Build history of the part. All positions in model axes, mm. A direction names the side the tool comes from. Coordinates: 2 decimals unless noted, no trailing zeros. Write each loop counter-clockwise with the first axis right and the second up, starting at its lowest first coordinate (ties: lowest second). Pieces come first, ordered by that corner, then holes.
Autodesk Inventor part; units mm, degrees
ref_plane "Work Plane1" through (29, 0, 0) normal (0, -1, 0) x (1, 0, 0)
ref_plane "YZ Plane" through (0, 0, 0) normal (1, 0, 0) x (0, 1, 0)
ref_plane "XZ Plane" through (0, 0, 0) normal (0, 1, 0) x (-1, 0, 0)
sketch "Эскиз1" plane through (0, 0, 0) normal (0, 0, 1) x (1, 0, 0)
  line L0 (-0.7333, 0) -> (16, 0)
  line L1 (16, 0) -> (16, 1.25)
  line L2 (16, 1.25) -> (1.35, 1.25)
  line L3 (1.35, 1.25) -> (1.0738, 1.25)
  line L4 (1.0738, 1.25) -> (0, 1.25)
  line L5 (0, 1.25) -> (0, 2.25)
  line L6 (0, 2.25) -> (-2.5, 2.25)
  line L7 (-2.5, 2.25) -> (-2.5, 1.1547)
  line L8 (-2.5, 1.1547) -> (-1.4, 1.1547)
  line L9 (-1.4, 1.1547) -> (-0.7333, 0)
  line L10 (-6.2, 0) -> (19.7, 0)
  line L11 (0, -0.45) -> (0, 2.7)
  line L12 (1.35, 1.25) -> (0, 1.25) construction
  dimension "d1" = 14.65
  dimension "d2" = 0.2762
  dimension "d3" = 2.5
  dimension "d4" = 1.1
  dimension "d5" = 60
  dimension "d6" = 2.5
  dimension "d7" = 2.5
  dimension "d8" = 2.3094
  dimension "d9" = 4.5
  dimension "d26" = 16
revolve "Базовый элемент" add sketch "Эскиз1" angle 360 about axis through (-0.7333, 0, 0) along (1, 0, 0)
sketch "Эскиз2" plane through (-2.5, 0, 0) normal (-1, 0, 0) x (0, 0, 1)
  circle A0 centre (0, 0) radius 1.1547
  line L0 (0, -3.15) -> (0, 3.15)
  line L1 (-3.15, 0) -> (3.15, 0)
  line L2 (1.1547, 0) -> (0.5774, -1)
  line L3 (0.5774, -1) -> (-0.5774, -1)
  line L4 (-0.5774, -1) -> (-1.1547, 0)
  line L5 (-1.1547, 0) -> (-0.5774, 1)
  line L6 (-0.5774, 1) -> (0.5774, 1)
  line L7 (0.5774, 1) -> (1.1547, 0)
extrude "Паз" add sketch "Эскиз2" against normal up to next contours L7 A0 | A0 L2 | L6 L0 A0 | A0 L0 L3 | L0 L6 A0 | A0 L3 L0 | L4 A0 | A0 L5
fillet "Сопряжение1" radius 0.25 1 edges at (-2.5, -2.25, 0)
thread "Резьба"
chamfer "Фаска1" distance 0.2761 distance2 0.2761 1 edges at (16, -1.25, 0) measured on face at (16, -0.3871, -0.3429)
ref_plane "Work Plane1" through (29, 0, 0) normal (0, -1, 0) x (1, 0, 0)
fillet "Fillet2" radius 0.1 1 edges at (0, -1.25, 0)
equation "\"d1\" = GEL"
equation "\"d3\" = KOH"
equation "\"d4\" = INTI"
equation "\"d6\" = GD"
equation "\"d7\" = BDM"
equation "\"d8\" = 1.1547 * SW"
equation "\"d9\" = KOD"
equation "\"d26\" = NLG"
equation "\"d30\" = R"
equation "\"d17\" = RR"
equation "\"d13\" = GEL"
equation "\"d15\" = -0.5 * SPD + 0.5 * GD"
equation "\"d16\" = GUL"
equation "\"GD\" = 2.5"
equation "\"NLG\" = 16"
equation "\"GEL\" = 14.65"
equation "\"KOD\" = 4.5"
equation "\"KOH\" = 2.5"
equation "\"INTI\" = 1.1"
equation "\"GAL\" = 0.61345 * PTC"
equation "\"GUL\" = 0.61345 * PTC"
equation "\"BDM\" = NND"
equation "\"SW\" = 2"
equation "\"RR\" = 0.25"
equation "\"SPD\" = NND - 1.2269 * PTC"
equation "\"R\" = 0.1"
equation "\"TOA\" = 30deg"
equation "\"GD1\" = THREADDIA - 1.2269 * PTC"
equation "\"THREADDIA\" = 2.5"
equation "\"FAWI\" = 45deg"
equation "\"PTC\" = 0.45"
equation "\"NND\" = 2.5"
equation "\"E0\" = 1.155 * SW"
properties part number "ISO 4762  - M2,5 x 16" material "Сталь нержавеющая, 440C"
(1) Slice it at A-A, the plane x = -0.5. List the corners of the cut face in (y, z).
(2) Two-plate mould, pull along Z, no slides. Class faces 4 (the flat face through (-2.5, -1, 1)), 5 (the conical face through (-0.775, 0.069, -0.022)), 6 (the flat face through (-2, 1, 0)), 7 (the cylindrical face through (7.8, -0.27, 1.22)): pulls with the +Z half, pulls with the -Z half, needs draft (parallel to the pull), parting line crosses it, or undercut.
(3) Slice it at B-B, the plane x = 1.5. List the corners of the cut face in (y, z), and give its area (3 significant figures).
(4) Probe L1, parallel to X at y = 1.5, z = -0.95; L2, parallel to Z at x = 9.75, y = 0.4; L3, parallel to Y at x = 8.75, z = -1. List the from-to ranges inside material, lowest first.
(5) Flat gauge pins, fed straight in: P1, Ø2, axis at x = 3.5, y = -1, coming from the +Z side; P2, Ø2, axis at x = 13.5, y = 0, coming from the -Z side; P3, Ø1.5, axis at x = 13, z = 0, coming from the -Y side. Where does each tip first touch, or does it go through?
(6) 3-axis set-ups, long thin cutter, end or side, ignore diameter. For faces 1 (the flat face through (-1.91, -0.51, -0.86)), 2 (the flat face through (0, 0.5, -1.5)), 3 (the cylindrical face through (-1.14, -0.29, -2.23)): which of +Z, -Z, +X, -X, +Y, -Y reach the whole face in a straight line?
Results:
1. outline: circle Ø4.5 at (0, 0)
2. face 4: needs draft
2. face 5: undercut
2. face 6: undercut
2. face 7: parting line crosses it
3. outline: circle Ø2.5 at (0, 0)
3. area: 4.91 mm2
4. L1: x = -2.5 to 0
4. L2: z = -1.18 to 1.18
4. L3: y = -0.75 to 0.75
5. P1: stops at z = 1.25
5. P2: stops at z = -1.25
5. P3: stops at y = -1.25
6. face 1: -X
6. face 2: +X
6. face 3: +X, -X
